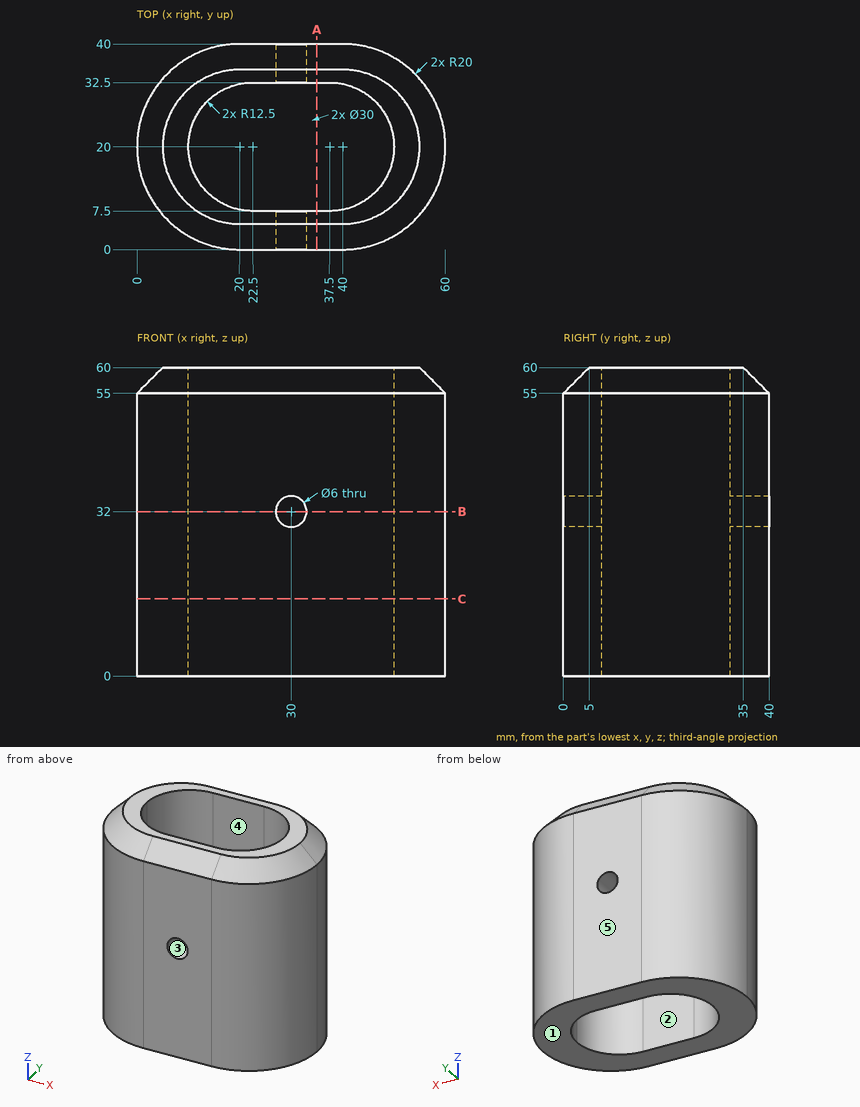
Job drawing, mm, ordinate dimensions from the low corner. One solid piece. A direction names the side the tool comes from. Give positions to 0.01 mm unless a question says otherwise; leave off trailing zeros. Order: outer loops, then holes, each group sorted by start corner. A loop starts at its lowest first (then second) coordinate and runs counter-clockwise, first axis right, second up. Notation, with made-up numbers: (8, 55) - (67, 55) arc R11 cw to (67, 76) - close; hole circle Ø11 at (-38.75, 14). An arc over 180 degrees is marked (long way). Return JSON: item names as keys, results as strings.
1) Cut at C-C, the plane z = 15. Give the cut face in (x, y), plus the area to 3 significant figures.
Geometry says:
{"outline": "(20, 0) - (40, 0) arc R20 ccw to (40, 40) - (20, 40) arc R20 ccw to start; hole (22.5, 7.5) - (37.5, 7.5) arc R12.5 ccw to (37.5, 32.5) - (22.5, 32.5) arc R12.5 ccw to start", "area": "1,190 mm²"}
2) Probe line 1 (Y direction, x = 26, z = 39.5); line 2 (Z direction, x = 30, y = 34); line 3 (Y direction, x = 12.5, z = 35). List the from-to ranges inside material, lowest first. Write a range as from..to.
Geometry says:
{"line 1": "0..7.5, 32.5..40", "line 2": "0..29, 35..60", "line 3": "1.46..12.5, 27.5..38.54"}
3) Cut at A-A, the plane x = 35. Give the cut face in (y, z).
Geometry says:
{"outline": "(0, 0) - (7.5, 0) - (7.5, 60) - (5, 60) - (0, 55) - close; (32.5, 0) - (40, 0) - (40, 55) - (35, 60) - (32.5, 60) - close"}
4) Flat gauge pins, fed straight in: P1, Ø1.5, axis at y = 21.5, z = 47.5, coming from the -X side; P2, Ø6, axis at x = 49.5, z = 32.5, coming from the +Y side; P3, Ø2, axis at y = 24.5, z = 6, coming from the +X side. Where does each tip first touch, or does it go through?
Geometry says:
{"P1": "x = 0.01", "P2": "y = 38.91", "P3": "x = 59.69"}
5) Cut at B-B, the plane z = 32. Give the cut face in (x, y), plus the area to 3 significant figures.
Geometry says:
{"outline": "(20, 0) - (27, 0) - (27, 7.5) - (22.5, 7.5) arc R12.5 cw to (22.5, 32.5) - (27, 32.5) - (27, 40) - (20, 40) arc R20 ccw to start; (33, 0) - (40, 0) arc R20 ccw to (40, 40) - (33, 40) - (33, 32.5) - (37.5, 32.5) arc R12.5 cw to (37.5, 7.5) - (33, 7.5) - close", "area": "1,100 mm²"}
6) Pull direction X, two halves, no side cores. Call the marked faces 1, 2 and 3: pulls with the +X half, pulls with the -X half, needs draft (parallel to the pull), parting line crosses it, or undercut.
Geometry says:
{"face 1": "needs draft", "face 2": "undercut", "face 3": "undercut"}
7) 3-axis set-ups, long thin cutter, end or side, ignore diameter. For the marked faces 4 and 5: which of +Z, -Z, +X, -X, +Y, -Y reach the whole face in a straight line?
Geometry says:
{"face 4": "+Z, -Z", "face 5": "+Z, -Z, +X, -X, +Y"}
